Can you work these out from the model? Positions are in its coordinate system, mm. A direction names the side the tool comes from. Round coordinates to 2 decimals unless told otherwise and drop trailing zeros. Order: outer loops, then holes, each group sorted by start corner. A loop starts at its lowest first (then second) coordinate and runs counter-clockwise, first axis right, second up. Notation, with made-up numbers: (41.25, -22) -> (64.25, -22) arc R38 cw to (64.25, 17) -> close; hole circle Ø11 at (2, 21.25). An arc over 180 degrees is marked (long way). Use a Markdown table: item, result. Add a question column.
Q1. We'd pull the mould along X, two halves only. Please class faces 5 (the face through (28.577, -21.596, -11.3)), 6 (the face through (-28.57, -21.6, -11.43)), 7 (the face through (0.244, -9.817, 4.156)), 8 (the face through (26.73, -0.043, 0.683)): +X half, -X half, draft (parallel to the pull), parting line (faces both ways), or undercut.
Q2. For faces 1 (the face through (24, -13, -6.74)), 2 (the face through (30.003, -10, -11)), 3 (the face through (-29.997, -10, -11)), 4 (the face through (-17.49, -13, 4)), which set-ups out of +Z, -Z, +X, -X, +Y, -Y let a thin tool reach every point of the face, with its end or its side?
Q3. If we section it at D-D on x = -20.5: List the corners of the cut face in (y, z) for me, plus the area to 3 significant figures.
Q4. If we section it at C-C on z = -11: List the corners of the cut face in (x, y) for me, plus the area to 3 significant figures.
Q5. If we section it at A-A on z = 2.5: List the corners of the cut face in (x, y) for me, plus the area to 3 significant figures.
Q6. I'm going to push flat-ended pins straight in: pin 1 Ø10 at (y, z) = (-9, -11.5) entering from -X; pin 2 Ø6.5 at (x, y) = (-21, -16.5) entering from +Z; pin 3 Ø10 at (y, z) = (-10.5, -13.5) entering from +X. Where does each tip first touch, or does it pass through?
Q7. I need wall thicknesses on line 1 along Z through (x, y) = (-25, 1.5); line 2 along Z through (x, y) = (-23.5, -5); line 3 along X through (y, z) = (-4.5, 2). Which ranges of each line are inside material? Lowest first, please. Write a range as [from, to].
Q8. If we section it at B-B on y = -14.5: List the corners of the cut face in (x, z) for me (3 decimals), plus the area to 3 significant figures.
```python
from build123d import *

# Parameters (mm, degrees)
F1_DEPTH = 3.1
F3_DEPTH = 20
F4_R     = 5
F5_R     = 3.75
F6_DEPTH = 25.4


with BuildPart() as f1:
    # F0 (on Front) → F1 (new body, symmetric)
    with BuildSketch(Plane.XZ):
        with BuildLine():
            Line((-35.43221, 15.260131), (-35.43221, -15.989869))
            Line((-35.43221, -15.989869), (35.06779, -15.989869))
            Line((35.06779, -15.989869), (35.06779, 15.260131))
            Line((35.06779, 15.260131), (11.124986, 15.260131))
            ThreePointArc((11.124986, 15.260131), (0, 4.152949), (-11.124986, 15.260131))
            Line((-11.124986, 15.260131), (-35.43221, 15.260131))
        make_face()
    extrude(amount=F1_DEPTH, both=True)

    # F2 (on face) → F3 (join)
    with BuildSketch(Plane.XZ.offset(3.1)):
        with BuildLine():
            Line((-11.124986, 15.260131), (-17.490178, 15.260131))
            Line((-17.490178, 15.260131), (-17.490178, -6.739869))
            Line((-17.490178, -6.739869), (-29.9974, -6.739869))
            Line((-29.9974, -6.739869), (-29.9974, -15.989869))
            Line((-29.9974, -15.989869), (30.0026, -15.989869))
            Line((30.0026, -15.989869), (30.0026, -6.739869))
            Line((30.0026, -6.739869), (17.509822, -6.739869))
            Line((17.509822, -6.739869), (17.509822, 15.260131))
            Line((17.509822, 15.260131), (11.124986, 15.260131))
            ThreePointArc((11.124986, 15.260131), (0, 4.152949), (-11.124986, 15.260131))
        make_face()
    extrude(amount=F3_DEPTH)

    # F4
    f4_edges = [f1.edges().sort_by_distance(p)[0] for p in [
        (-29.9974, -23.1, -11.364869),
        (30.0026, -23.1, -11.364869),
    ]]
    fillet(f4_edges, radius=F4_R)

    # F5 (on face) → F6 (cut)
    with BuildSketch(Plane.XZ.offset(3.1)):
        with Locations((-25, 4.010131)):
            Circle(F5_R)
        with Locations((25, 4.010131)):
            Circle(F5_R)
    extrude(amount=-F6_DEPTH, mode=Mode.SUBTRACT)


solid = f1.part
```
Answer below:
| question | item | result |
|---|---|---|
| 1 | face 5 | +X half |
| 1 | face 6 | -X half |
| 1 | face 7 | undercut |
| 1 | face 8 | undercut |
| 2 | face 1 | +Z, +X, -Y |
| 2 | face 2 | +Z, -Z, +X, -Y |
| 2 | face 3 | +Z, -Z, -X, -Y |
| 2 | face 4 | +Z, -X, -Y |
| 3 | outline | (-23.1, -15.99) -> (3.1, -15.99) -> (3.1, 15.26) -> (-3.1, 15.26) -> (-3.1, -6.74) -> (-23.1, -6.74) -> close |
| 3 | area | 379 mm² |
| 4 | outline | (-35.43, -3.1) -> (-30, -3.1) -> (-30, -18.1) arc R5 ccw to (-25, -23.1) -> (25, -23.1) arc R5 ccw to (30, -18.1) -> (30, -3.1) -> (35.07, -3.1) -> (35.07, 3.1) -> (-35.43, 3.1) -> close |
| 4 | area | 1,630 mm² |
| 5 | outline | (-35.43, -3.1) -> (-28.43, -3.1) -> (-28.43, 3.1) -> (-35.43, 3.1) -> close; (-21.57, -3.1) -> (-17.49, -3.1) -> (-17.49, -23.1) -> (17.51, -23.1) -> (17.51, -3.1) -> (21.57, -3.1) -> (21.57, 3.1) -> (-21.57, 3.1) -> close; (28.43, -3.1) -> (35.07, -3.1) -> (35.07, 3.1) -> (28.43, 3.1) -> close |
| 5 | area | 1,050 mm² |
| 6 | pin 1 | x = -30 |
| 6 | pin 2 | z = -6.74 |
| 6 | pin 3 | x = 30 |
| 7 | line 1 | [-15.99, 0.26], [7.76, 15.26] |
| 7 | line 2 | [-15.99, -6.74] |
| 7 | line 3 | [-17.49, 17.51] |
| 8 | outline | (-29.997, -15.99) -> (30.003, -15.99) -> (30.003, -6.74) -> (17.51, -6.74) -> (17.51, 15.26) -> (11.125, 15.26) arc R11.125 cw to (-11.125, 15.26) -> (-17.49, 15.26) -> (-17.49, -6.74) -> (-29.997, -6.74) -> close |
| 8 | area | 1,130 mm² |
